from build123d import *

# Parameters (mm, degrees)
F0_R     = 8
F1_DEPTH = 3.5
F2_DEPTH = 4.5
F4_DEPTH = 1.5


with BuildPart() as f1:
    # F0 (on Top) → F1 (new body)
    with BuildSketch(Plane.XY):
        with BuildLine():
            ThreePointArc((0, -12.5), (8.838835, -8.838835), (12.5, 0))
            ThreePointArc((12.5, 0), (8.838835, 8.838835), (0, 12.5))
            ThreePointArc((0, 12.5), (-12.5, 0), (0, -12.5))
        make_face()
        Circle(F0_R, mode=Mode.SUBTRACT)
        with BuildLine():
            ThreePointArc((0, 12.5), (8.838835, 8.838835), (12.5, 0))
            ThreePointArc((12.5, 0), (8.838835, -8.838835), (0, -12.5))
            Line((0, -12.5), (35, -12.5))
            Line((35, -12.5), (116.388784, -2.506714))
            Line((116.388784, -2.506714), (116.388784, 2.506714))
            Line((116.388784, 2.506714), (35, 12.5))
            Line((35, 12.5), (0, 12.5))
        make_face()
    extrude(amount=F1_DEPTH)

    # F0 (on Top) → F2 (join)
    with BuildSketch(Plane.XY):
        with BuildLine():
            ThreePointArc((0, -12.5), (8.838835, -8.838835), (12.5, 0))
            ThreePointArc((12.5, 0), (8.838835, 8.838835), (0, 12.5))
            ThreePointArc((0, 12.5), (-12.5, 0), (0, -12.5))
        make_face()
        Circle(F0_R, mode=Mode.SUBTRACT)
    extrude(amount=F2_DEPTH)

    # F3 (on face) → F4 (cut)
    with BuildSketch(Plane.XY.offset(3.5)):
        Polygon((116.388784, 0), (116.388784, 1.006714), (96.388784, 1.006714), (96.388784, 0), (96.388784, -0.993286), (116.388784, -0.993286), align=None)
    extrude(amount=-F4_DEPTH, mode=Mode.SUBTRACT)


solid = f1.part
For this review, take the finished solid that the model builds, in its own axes (mm). Give positions to 0.01 mm unless a question says otherwise; leave off trailing zeros. Loops run counter-clockwise (first coordinate to the right, second up) from the corner with the lowest first, then second, coordinate; pieces in that order, holes last.
Item 1: Take a section at D-D, the plane x = 80.5. State the section outline as (y, z) points, and give its area (3 significant figures).
Item 2: Take a section at C-C, the plane y = 9.25. State the section outline as (x, z) points, and give its area (3 significant figures).
Item 3: For line 1 along Y through (x, z) = (0, 1.6); line 2 along X through (y, z) = (-0.5, 1.5); line 3 along X through (y, z) = (0.5, 3.3), list the stretches that pass through material, from the lowest coordinate up.
Item 4: Insertion check: pin 1 (1.2 mm diameter, centred on x = 103.5, z = 2.5, fed in from +Y); pin 2 (7.5 mm diameter, centred on x = 46.5, y = -2, fed in from +Z); pin 3 (2 mm diameter, centred on x = 41.5, z = 3.5, fed in from +Y). Each pin has a flat end and moves straight along its axis. Give the tip position at first contact, or say it passes through.
Item 5: Take a section at B-B, the plane x = 102.5. State the section outline as (y, z) points, and give its area (3 significant figures).
Item 6: Take a section at A-A, the plane y = -5. State the section outline as (x, z) points (3 decimals).
Item 7: Draft analysis for pull direction X (two halves, no side actions). For faces 1 (the cylindrical face through (-1.73, -7.81, 2.22)), 2 (the flat face through (106, 0, 2)), 3 (the flat face through (116.389, 0, 1.7)), state which applies: +X half, -X half, draft (parallel to the pull), parting line (faces both ways), or undercut.
Calculated:
1. outline: (-6.91, 0) - (6.91, 0) - (6.91, 3.5) - (-6.91, 3.5) - close
1. area: 48.4 mm2
2. outline: (-8.41, 0) - (61.47, 0) - (61.47, 3.5) - (8.41, 3.5) - (8.41, 4.5) - (-8.41, 4.5) - close
2. area: 261 mm2
3. line 1: y = -12.5 to -8, 8 to 12.5
3. line 2: x = -12.49 to -7.98, 7.98 to 116.39
3. line 3: x = -12.49 to -7.98, 7.98 to 96.39
4. pin 1: stops at y = 4.16
4. pin 2: stops at z = 3.5
4. pin 3: stops at y = 11.82
5. outline: (-4.21, 0) - (4.21, 0) - (4.21, 3.5) - (1.01, 3.5) - (1.01, 2) - (-0.99, 2) - (-0.99, 3.5) - (-4.21, 3.5) - close
5. area: 26.5 mm2
6. outline: (-11.456, 0) - (-6.245, 0) - (-6.245, 4.5) - (-11.456, 4.5) - close; (6.245, 0) - (96.083, 0) - (96.083, 3.5) - (11.456, 3.5) - (11.456, 4.5) - (6.245, 4.5) - close
7. face 1: undercut
7. face 2: draft
7. face 3: +X half
